Geometry: final body of the model. Coordinates: model frame, mm. Round coordinates to 2 decimals unless told otherwise and drop trailing zeros. Loops run counter-clockwise (first coordinate to the right, second up) from the corner with the lowest first, then second, coordinate; pieces in that order, holes last. Notation, with made-up numbers: (74.5, 61.25) - (88.5, 61.25) arc R10 cw to (88.5, 78.25) - close; hole circle Ø8 at (56.25, 71.5). An arc over 180 degrees is marked (long way). Answer as a JSON object with one key per item and string values. Group by question number.
Item 1: Line query: line 1 (X direction, y = 2.5, z = 1.2); line 2 (Z direction, x = 22.5, y = -20.5); line 3 (Z direction, x = 25.5, y = -18.5). Output: solid intervals per line, ascending.
Item 2: Section B-B (x = 20.5). Return the cut outline in (y, z).
Item 3: Section C-C (y = 2). Return the cut outline in (x, z).
Item 4: Section A-A (y = -19). Return the cut outline in (x, z), plus the area to 3 significant figures.
Item 5: First-contact query: pin 1 (3 mm diameter, centred on x = -47, y = -18.5, fed in from -Z); pin 2 (4 mm diameter, centred on x = 33.5, y = 18.5, fed in from +Z); pin 3 (0.8 mm diameter, centred on x = -15.5, z = 1.5, fed in from +Y); pin 4 (0.8 mm diameter, centred on y = -4, z = 1.5, fed in from -X). Flat tips, straight axial feed; report the tip coordinate or a pass-through.
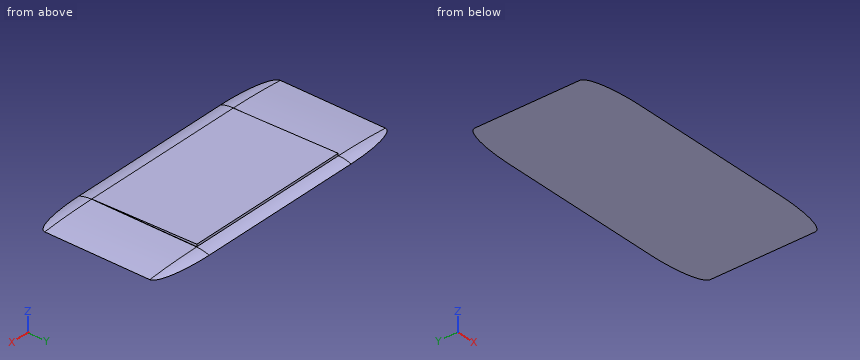
```python
from build123d import *

# Parameters (mm, degrees)
F0_W         = 120
F0_H         = 75
F1_DEPTH     = 1
F0_W_2       = 24
F0_H_2       = 45
F2_DEPTH     = 2
F3_DEPTH     = 2
F4_DEPTH     = 2
F6_DEPTH     = 1000
F7_T1_DEPTH  = 194.2686044191
F8_T1_DEPTH  = 194.2686044191
F9_T1_DEPTH  = 72.2925582324
F9_T4_ANGLE  = 12.3400437426
F9_T6_ANGLE  = 12.3400437426
F10_T1_DEPTH = 72.2925582324
F10_T4_ANGLE = 12.3400437426
F10_T6_ANGLE = 12.3400437426


# Not quite as in the source:
# - a fillet or chamfer that OpenCascade refuses, or shapes differently, is made with other operations: its cross-section is extruded or revolved along the edge and cut away or added


with BuildPart() as f1:
    # F0 (on Top) → F1 (new body)
    with BuildSketch(Plane.XY):
        Rectangle(F0_W, F0_H)
        Polygon((-36, -22.5), (-36, 22.5), (-12, 22.5), (12, 22.5), (36, 22.5), (36, -22.5), (12, -22.5), (-12, -22.5), align=None, mode=Mode.SUBTRACT)
    extrude(amount=F1_DEPTH)

    # F0 (on Top) → F2 (join)
    with BuildSketch(Plane.XY):
        with Locations((-24, 0)):
            Rectangle(F0_W_2, F0_H_2)
    extrude(amount=F2_DEPTH)

    # F0 (on Top) → F3 (join)
    with BuildSketch(Plane.XY):
        Rectangle(F0_W_2, F0_H_2)
    extrude(amount=F3_DEPTH)

    # F0 (on Top) → F4 (join)
    with BuildSketch(Plane.XY):
        with Locations((24, 0)):
            Rectangle(F0_W_2, F0_H_2)
    extrude(amount=F4_DEPTH)

    # F5 (on face) → F6 (cut)
    with BuildSketch(Plane(origin=(-60, 0, 0), x_dir=(0, -1, 0), z_dir=(-1, 0, 0))):
        Polygon((22.5, 2), (-22.5, 2), (22.5, 1), align=None)
    extrude(amount=-F6_DEPTH, mode=Mode.SUBTRACT)

    # F7: fillet of radius 285 on 1 edges, made by hand

    # F7_s2 → F7_t1 (cut)
    with BuildSketch(Plane.XZ.offset(-97.1343022095)):
        with BuildLine():
            ThreePointArc((-36.1462791162, 1), (-48.0836155025, 0.7498902546), (-60, 0))
            Line((-60, 0), (-60, 1))
            Line((-60, 1), (-36.1462791162, 1))
        make_face()
    extrude(amount=F7_T1_DEPTH, mode=Mode.SUBTRACT)

    # F8: fillet of radius 285 on 1 edges, made by hand

    # F8_s2 → F8_t1 (cut)
    with BuildSketch(Plane.XZ.offset(-97.1343022095)):
        with BuildLine():
            ThreePointArc((36.1462791162, 1), (48.0836155025, 0.7498902546), (60, 0))
            Line((60, 0), (60, 1))
            Line((60, 1), (36.1462791162, 1))
        make_face()
    extrude(amount=F8_T1_DEPTH, mode=Mode.SUBTRACT)

    # F9: fillet of radius 15 on 1 edges, made by hand

    # F9_s2 → F9_t1 (cut)
    with BuildSketch(Plane.YZ.offset(-36.1462791162)):
        with BuildLine():
            ThreePointArc((-22.5, 1), (-33.1066017178, -3.3933982822), (-37.5, -14))
            Line((-37.5, -14), (-37.5, 1))
            Line((-37.5, 1), (-22.5, 1))
        make_face()
    extrude(amount=F9_T1_DEPTH, mode=Mode.SUBTRACT)

    # F9_s3 → F9_t4 (revolve, cut)
    with BuildSketch(Plane(origin=(-93.7876438564, 0, -20.5176876571), x_dir=(0, 1, 0), z_dir=(-0.9768964499, 0, -0.2137131866))):
        with BuildLine():
            ThreePointArc((-22.5, -15.2863447158), (-33.1066017178, -10.8929464336), (-37.5, -0.2863447158))
            Line((-37.5, -0.2863447158), (-37.5, -15.2863447158))
            Line((-37.5, -15.2863447158), (-22.5, -15.2863447158))
        make_face()
    revolve(axis=Axis((-36.1462791167, -37.5, -283.9999999893), (0, 1, 0)), revolution_arc=F9_T4_ANGLE, mode=Mode.SUBTRACT)

    # F9_s5 → F9_t6 (revolve, cut)
    with BuildSketch(Plane.YZ.offset(36.1462791167)):
        with BuildLine():
            ThreePointArc((-22.5, 1), (-33.1066017178, -3.3933982822), (-37.5, -14))
            Line((-37.5, -14), (-37.5, 1))
            Line((-37.5, 1), (-22.5, 1))
        make_face()
    revolve(axis=Axis((36.1462791167, -37.5, -283.9999999893), (0, 1, 0)), revolution_arc=F9_T6_ANGLE, mode=Mode.SUBTRACT)

    # F10: fillet of radius 15 on 1 edges, made by hand

    # F10_s2 → F10_t1 (cut)
    with BuildSketch(Plane.YZ.offset(-36.1462791162)):
        with BuildLine():
            ThreePointArc((37.5, -14), (33.1066017178, -3.3933982822), (22.5, 1))
            Line((22.5, 1), (37.5, 1))
            Line((37.5, 1), (37.5, -14))
        make_face()
    extrude(amount=F10_T1_DEPTH, mode=Mode.SUBTRACT)

    # F10_s3 → F10_t4 (revolve, cut)
    with BuildSketch(Plane.YZ.offset(36.1462791167)):
        with BuildLine():
            ThreePointArc((37.5, -14), (33.1066017178, -3.3933982822), (22.5, 1))
            Line((22.5, 1), (37.5, 1))
            Line((37.5, 1), (37.5, -14))
        make_face()
    revolve(axis=Axis((36.1462791167, 37.5, -283.9999999893), (0, 1, 0)), revolution_arc=F10_T4_ANGLE, mode=Mode.SUBTRACT)

    # F10_s5 → F10_t6 (revolve, cut)
    with BuildSketch(Plane(origin=(-93.7876438564, 0, -20.5176876571), x_dir=(0, 1, 0), z_dir=(-0.9768964499, 0, -0.2137131866))):
        with BuildLine():
            ThreePointArc((37.5, -0.2863447158), (33.1066017178, -10.8929464336), (22.5, -15.2863447158))
            Line((22.5, -15.2863447158), (37.5, -15.2863447158))
            Line((37.5, -15.2863447158), (37.5, -0.2863447158))
        make_face()
    revolve(axis=Axis((-36.1462791167, 37.5, -283.9999999893), (0, 1, 0)), revolution_arc=F10_T6_ANGLE, mode=Mode.SUBTRACT)


solid = f1.part
```
Values:
{
 "1": {"line 1": "x = -36 to 36", "line 2": "z = 0 to 1.04", "line 3": "z = 0 to 1.09"},
 "2": {"outline": "(-27.89, 0) - (27.89, 0) arc R15 ccw to (22.5, 1) - (22.5, 2) - (-22.5, 1) arc R15 ccw to start"},
 "3": {"outline": "(-60, 0) - (60, 0) arc R285 ccw to (36.15, 1) - (36, 1) - (36, 1.54) - (-36, 1.54) - (-36, 1) - (-36.15, 1) arc R285 ccw to start"},
 "4": {"outline": "(-60, 0) - (60, 0) arc R285 ccw to (36.15, 1) - (36, 1) - (36, 1.08) - (-36, 1.08) - (-36, 1) - (-36.15, 1) arc R285 ccw to start", "area": "110 mm^2"},
 "5": {"pin 1": "stops at z = 0", "pin 2": "stops at z = 1.96", "pin 3": "stops at y = 22.5", "pin 4": "stops at x = -36"}
}
